Autodesk Inventor part; units mm, degrees
ref_plane "YZ Plane" through (0, 0, 0) normal (1, 0, 0) x (0, 1, 0)
ref_plane "XZ Plane" through (0, 0, 0) normal (0, 1, 0) x (-1, 0, 0)
ref_plane "XY Plane" through (0, 0, 0) normal (0, 0, 1) x (1, 0, 0)
sketch "Sketch1" plane through (0, 0, 0) normal (0, 1, 0) x (-1, 0, 0)
  line L0 (-50.8, 114.3) -> (50.8, 114.3)
  line L1 (50.8, 114.3) -> (50.8, -114.3)
  line L2 (50.8, -114.3) -> (-50.8, -114.3)
  line L3 (-50.8, -114.3) -> (-50.8, 114.3)
  line L4 (-50.8, 114.3) -> (50.8, -114.3) construction
  line L5 (50.8, 114.3) -> (-50.8, -114.3) construction
  line L6 (-50.8, 88.9) -> (25.4, 88.9)
  line L7 (25.4, 88.9) -> (24.8543, -88.9)
  line L8 (24.8543, -88.9) -> (-50.8, -88.9)
  point P0 (0, 0)
  dimension "d0" = 101.6
  dimension "d1" = 228.6
  dimension "d2" = 76.2
  dimension "d3" = 25.4
  dimension "d4" = 25.4
extrude "Extrusion1" add sketch "Sketch1" along normal blind 38.1 contours L0 L1 L2 L3 L8 L7 L6
fillet "Fillet1" radius 12.7 4 edges at (50.8, 19.05, 114.3) (-50.8, 19.05, 114.3) (-50.8, 19.05, -114.3) (50.8, 19.05, -114.3)
sketch "Sketch2" plane through (0, 38.1, 0) normal (0, 1, 0) x (1, 0, 0)
  line L0 (-38.1, -114.3) -> (38.1, -114.3)
  circle A0 centre (-35.8052, -101.6) radius 3.3782
  line L1 (-35.8052, -101.6) -> (-35.8052, 101.6) construction
  line L2 (-35.8052, -101.6) -> (40.3948, -101.6) construction
  line L3 (-35.8052, 101.6) -> (40.3948, 101.6) construction
  circle A1 centre (-35.8052, -88.3158) radius 3.3782 construction
  line L4 (-39.1834, -98.2218) -> (-30.0963, -98.2218) construction
  circle A2 centre (-35.8052, -75.0316) radius 3.3782 construction
  circle A3 centre (-35.8052, -61.7474) radius 3.3782 construction
  circle A4 centre (-35.8052, -48.4632) radius 3.3782 construction
  circle A5 centre (-35.8052, -35.179) radius 3.3782 construction
  circle A6 centre (-35.8052, -21.8948) radius 3.3782 construction
  circle A7 centre (-35.8052, -8.6106) radius 3.3782 construction
  circle A8 centre (-35.8052, 4.6736) radius 3.3782 construction
  circle A9 centre (-35.8052, 17.9578) radius 3.3782 construction
  circle A10 centre (-35.8052, 31.242) radius 3.3782 construction
  circle A11 centre (-35.8052, 44.5262) radius 3.3782 construction
  circle A12 centre (-35.8052, 57.8104) radius 3.3782 construction
  circle A13 centre (-35.8052, 71.0946) radius 3.3782 construction
  circle A14 centre (-35.8052, 84.3788) radius 3.3782 construction
  circle A15 centre (-35.8052, 97.663) radius 3.3782 construction
  circle A16 centre (-22.521, -101.6) radius 3.3782 construction
  circle A17 centre (-9.2368, -101.6) radius 3.3782 construction
  circle A18 centre (4.0474, -101.6) radius 3.3782 construction
  circle A19 centre (17.3316, -101.6) radius 3.3782 construction
  circle A20 centre (30.6158, -101.6) radius 3.3782 construction
  circle A21 centre (43.9, -101.6) radius 3.3782 construction
  circle A22 centre (30.6158, 97.663) radius 3.3782 construction
  circle A23 centre (30.6158, -101.6) radius 3.3782 construction
  circle A24 centre (-35.8052, 97.663) radius 3.3782 construction
  circle A25 centre (-35.8052, 31.242) radius 3.3782 construction
  circle A26 centre (-35.8052, -35.179) radius 3.3782 construction
  circle A27 centre (-35.8052, -35.179) radius 3.3782
  circle A28 centre (-35.8052, 31.242) radius 3.3782
  circle A29 centre (-35.8052, 97.663) radius 3.3782
  circle A30 centre (30.6158, 97.663) radius 3.3782
  circle A31 centre (30.6158, -101.6) radius 3.3782
  point P0 (0, 0)
  point P1 (-35.8052, -25.4)
  point P2 (-35.8052, 25.4)
  dimension "d8" = 12.7
  dimension "d9" = 76.2
  dimension "d10" = 127
  dimension "d11" = 203.2
  dimension "d12" = 76.2
  dimension "d13" = 6.7564
  dimension "d22" = 13.2842
  dimension "d25" = 13.2842
  dimension "d30" = 13.2842
  dimension "d33" = 13.2842
  dimension "d38" = 6.7564
  dimension "d39" = 6.7564
  dimension "d40" = 6.7564
  dimension "d41" = 6.7564
  dimension "d42" = 6.7564
  dimension "d43" = 6.7564
  dimension "d44" = 6.7564
  dimension "d45" = 6.7564
  dimension "d46" = 6.7564
extrude "Extrusion4" cut sketch "Sketch2" against normal through all
equation "\"d25\" = d22"
equation "\"d30\" = d22"
equation "\"d33\" = d22"
properties part number "FINALBH"
CAD build for the part. Positions are in the model's coordinates, mm. Give positions to 0.01 mm unless a question says otherwise; leave off trailing zeros. Write each loop counter-clockwise with the first axis right and the second up, starting at its lowest first coordinate (ties: lowest second). Pieces come first, ordered by that corner, then holes. Notation, with made-up numbers: M 76,-38 L 89,-38 A20 ccw 89,-17 Z; hole C -13.5,64.5 d4. An arc over 180 degrees is marked long. Put each result on its own line as item: value. Start each with the question number.
(1) Band-saw the part on A-A, the plane x = 17.5. Write the cut outline in (y, z).
(2) Band-saw the part on D-D, the plane z = 69.5. Write the cut outline in (x, y).
(3) Probe L1, parallel to X at y = 13.5, z = 101.6; L2, parallel to Z at x = 6, y = 25; L3, parallel to Z at x = 32.5, y = 5.5. List the from-to ranges inside material, lowest first.
(4) Mould opens along Z. For faces 1 (the face through (28.126, 19.317, 99.317)), 2 (the face through (-50.8, 19, 1)), 3 (the face through (-47.18, 19.32, 110.48)), 4 (the face through (12, 19, -88.9)) say: +Z half, -Z half, draft (parallel to the pull), parting line (faces both ways), or undercut.
(5) Band-saw the part on C-C, the plane y = 20. Write the cut outline in (x, z).
(6) Flat gauge pins, fed straight in: pin 1 Ø1.5 at (y, z) = (29, 73.5) entering from +X; pin 2 Ø6 at (y, z) = (26.5, -13) entering from +X. Where does each tip first touch, or does it go through?
(7) Band-saw the part on B-B, the plane x = -36. Write the cut outline in (y, z).
Response values:
1. outline: M 0,-114.3 L 38.1,-114.3 L 38.1,-88.9 L 0,-88.9 Z; M 0,88.9 L 38.1,88.9 L 38.1,114.3 L 0,114.3 Z
2. outline: M -50.8,0 L -25.34,0 L -25.34,38.1 L -50.8,38.1 Z
3. L1: x = -50.8 to -39.18, -32.43 to 27.24, 33.99 to 50.8
3. L2: z = -114.3 to -88.9, 88.9 to 114.3
3. L3: z = -114.3 to -100.47, -94.86 to -88.9, 88.9 to 98.8, 104.4 to 114.3
4. face 1: undercut
4. face 2: draft
4. face 3: +Z half
4. face 4: undercut
5. outline: M -50.8,-101.6 A12.7 ccw -38.1,-114.3 L 38.1,-114.3 A12.7 ccw 50.8,-101.6 L 50.8,-88.9 L -24.85,-88.9 L -25.4,88.9 L 50.8,88.9 L 50.8,101.6 A12.7 ccw 38.1,114.3 L -38.1,114.3 A12.7 ccw -50.8,101.6 Z; hole C -35.81,-97.66 d6.76; hole C -35.81,-31.24 d6.76; hole C -35.81,35.18 d6.76; hole C -35.81,101.6 d6.76; hole C 30.62,-97.66 d6.76; hole C 30.62,101.6 d6.76
6. pin 1: stops at x = -25.35
6. pin 2: stops at x = -25.08
7. outline: M 0,-114.3 L 38.1,-114.3 L 38.1,-101.04 L 0,-101.04 Z; M 0,-94.29 L 38.1,-94.29 L 38.1,-34.61 L 0,-34.61 Z; M 0,-27.87 L 38.1,-27.87 L 38.1,31.81 L 0,31.81 Z; M 0,38.55 L 38.1,38.55 L 38.1,98.23 L 0,98.23 Z; M 0,104.97 L 38.1,104.97 L 38.1,114.3 L 0,114.3 Z
